```python
from build123d import *

# Parameters (mm, degrees)
CUT_EXTRUDE_1_DEPTH = 2
SCALE_1_SCALE       = 0.58


with BuildPart() as part:
    # 草图1 → 旋转1 (revolve)
    with BuildSketch(Plane.XY):
        Polygon((1.5, 70), (1.5, 72), (0, 72), (0, 70), (0, -3), (3.5, -3), (3.5, 0), (1.5, 0), align=None)
    revolve(axis=Axis((0, 78.762815816, 0), (0, -1, 0)))

    # 草图2 → 切除-拉伸1 (cut)
    with BuildSketch(Plane.XZ.offset(3)):
        Polygon((2.503979876, 0), (1.251989938, 2.168510183), (-1.251989938, 2.168510183), (-2.503979876, 0), (-1.251989938, -2.168510183), (1.251989938, -2.168510183), align=None)
    extrude(amount=-CUT_EXTRUDE_1_DEPTH, mode=Mode.SUBTRACT)


with BuildPart() as part_1:
    # 缩放比例1: scaled about (0, 30.776232498, 0)
    add(part.part.scale(SCALE_1_SCALE).moved(Location((0, 12.926017649, 0))))


solid = part_1.part
```
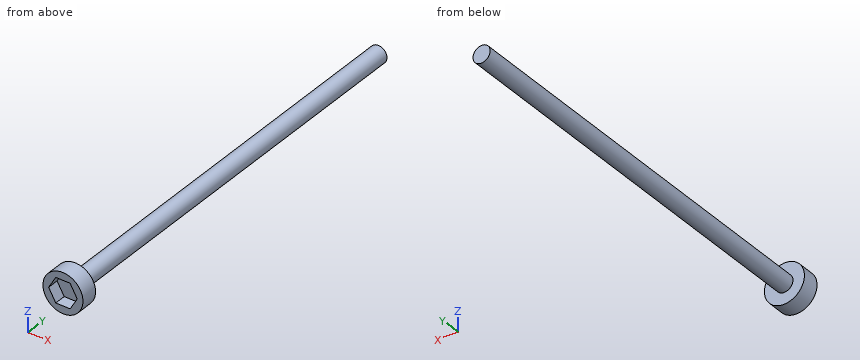
Here's how the part is built. I have some questions about the finished solid (model axes, mm). Round coordinates to 2 decimals unless told otherwise and drop trailing zeros. Loops run counter-clockwise (first coordinate to the right, second up) from the corner with the lowest first, then second, coordinate; pieces in that order, holes last. Notation, with made-up numbers: (5.5, 55.5) -> (22.5, 55.5) arc R30 ccw to (22.5, 89.5) -> close; hole circle Ø1 at (50, 15.5). An arc over 180 degrees is marked (long way). Answer as CSV lines item,"result". Start each with the question number.
1. Imagine slicing it at B-B on y = 38. Write out the boundary of the cut face in (x, z), plus the area to 3 significant figures.
2. I'm going to push flat-ended pins straight in: P1, Ø2, axis at y = 21.5, z = -0.5, coming from the +X side; P2, Ø1.5, axis at x = -0.5, y = 17.5, coming from the -Z side; P3, Ø2, axis at x = -1, y = 17.5, coming from the +Z side. Where does each tip first touch, or does it pass through?
3. Imagine slicing it at A-A on x = 0. Write out the boundary of the cut face in (y, z).
4. I need wall thicknesses on probe 1 along Y at (x, z) = (1.1, 0.25); probe 2 along Y at (x, z) = (-0.1, -0.6); probe 3 along X at (y, z) = (37.5, -0.05). Which ranges of each line are inside material? Lowest first, please. Write a range as from..to.
Solution:
1,outline,"circle Ø1.74 at (0, 0)"
1,area,"2.38 mm²"
2,P1,"x = 0.87"
2,P2,"z = -0.87"
2,P3,"z = 0.87"
3,outline,"(11.19, -2.03) -> (12.93, -2.03) -> (12.93, -0.87) -> (54.69, -0.87) -> (54.69, 0.87) -> (12.93, 0.87) -> (12.93, 2.03) -> (11.19, 2.03) -> (11.19, 1.26) -> (12.35, 1.26) -> (12.35, -1.26) -> (11.19, -1.26) -> close"
4,probe 1,"12.35..12.93"
4,probe 2,"12.35..54.69"
4,probe 3,"-0.87..0.87"
